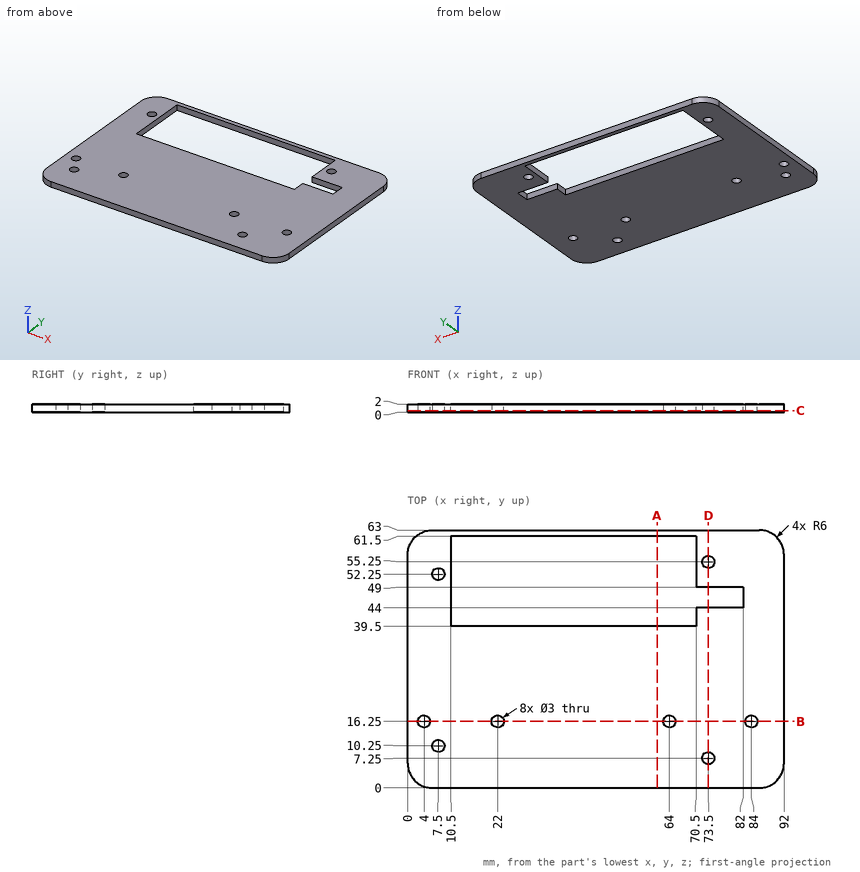
Print and shaded views of the part. All mm, measured from the part's lowest x, y and z. Round coordinates to 2 decimals unless told otherwise and drop trailing zeros. Write each loop counter-clockwise with the first axis right and the second up, starting at its lowest first coordinate (ties: lowest second). Pieces come first, ordered by that corner, then holes. Notation, with made-up numbers: (-14, 87) -> (44, 87) arc R22 ccw to (44, 123) -> close; hole circle Ø6 at (80.5, 23.25). An arc over 180 degrees is marked (long way). Return JSON: item names as keys, results as strings. Group by question number.
Q1. Probe L1, parallel to Y at x = 7.5, z = 1.4; L2, parallel to X at y = 55.25, z = 1.6; L3, parallel to Y at x = 73.5, z = 0.7. List the from-to ranges inside material, lowest first. Write a range as [from, to].
Q2. Saw through at B-B on y = 16.25. Write the cut outline in (x, z).
Q3. Saw through at C-C on z = 0.4. State how many separate pieces and enclosed holes the cut face has, plus the area to 3 significant figures.
Q4. Saw through at D-D on x = 73.5. Write the cut outline in (y, z), plus the area to 3 significant figures.
Q5. Saw through at A-A on x = 61. Write the cut outline in (y, z).
Answer:
{
 "1": {"L1": "[0, 8.75], [11.75, 50.75], [53.75, 63]", "L2": "[0, 10.5], [70.5, 72], [75, 92]", "L3": "[0, 5.75], [8.75, 44], [49, 53.75], [56.75, 63]"},
 "2": {"outline": "(0, 0) -> (2.5, 0) -> (2.5, 2) -> (0, 2) -> close; (5.5, 0) -> (20.5, 0) -> (20.5, 2) -> (5.5, 2) -> close; (23.5, 0) -> (62.5, 0) -> (62.5, 2) -> (23.5, 2) -> close; (65.5, 0) -> (82.5, 0) -> (82.5, 2) -> (65.5, 2) -> close; (85.5, 0) -> (92, 0) -> (92, 2) -> (85.5, 2) -> close"},
 "3": {"separate pieces": "1", "enclosed holes": "9", "area": "4,330 mm2"},
 "4": {"outline": "(0, 0) -> (5.75, 0) -> (5.75, 2) -> (0, 2) -> close; (8.75, 0) -> (44, 0) -> (44, 2) -> (8.75, 2) -> close; (49, 0) -> (53.75, 0) -> (53.75, 2) -> (49, 2) -> close; (56.75, 0) -> (63, 0) -> (63, 2) -> (56.75, 2) -> close", "area": "104 mm2"},
 "5": {"outline": "(0, 0) -> (39.5, 0) -> (39.5, 2) -> (0, 2) -> close; (61.5, 0) -> (63, 0) -> (63, 2) -> (61.5, 2) -> close"}
}
